Geometry check sheet. Reference: the model listing, model coordinates, mm. Face numbers are marked on the shaded views. A direction names the side the tool comes from. Round coordinates to 2 decimals unless told otherwise and drop trailing zeros. Write each loop counter-clockwise with the first axis right and the second up, starting at its lowest first coordinate (ties: lowest second). Pieces come first, ordered by that corner, then holes. Notation, with made-up numbers: (-34.5, 61.25) - (-22.5, 61.25) arc R15 ccw to (-22.5, 79.25) - close; hole circle Ø8 at (13, 28.25). An arc over 180 degrees is marked (long way). Return JSON: item names as keys, results as strings.
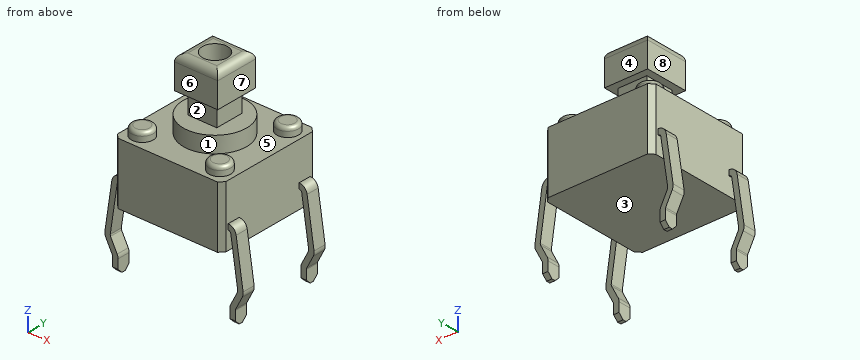
Autodesk Inventor part; units mm, degrees
ref_plane "YZ Plane" through (0, 0, 0) normal (1, 0, 0) x (0, 1, 0)
ref_plane "XZ Plane" through (0, 0, 0) normal (0, 1, 0) x (-1, 0, 0)
ref_plane "XY Plane" through (0, 0, 0) normal (0, 0, 1) x (1, 0, 0)
sketch "Sketch1" plane through (0, 0, 0) normal (0, 0, 1) x (1, 0, 0)
  line L0 (-2.75, -3) -> (2.75, -3)
  line L1 (3, -2.75) -> (3, 2.75)
  line L2 (2.75, 3) -> (-2.75, 3)
  line L3 (-3, 2.75) -> (-3, -2.75)
  line L4 (-3, -3) -> (3, 3) construction
  line L5 (3, -3) -> (-3, 3) construction
  line L6 (-2.75, 3) -> (-3, 2.75)
  line L7 (-3, -2.75) -> (-2.75, -3)
  line L8 (2.75, -3) -> (3, -2.75)
  line L9 (3, 2.75) -> (2.75, 3)
  point P0 (0, 0)
  dimension "d0" = 6
  dimension "d1" = 0.25
  dimension "d2" = 0.25
  dimension "d3" = 0.25
  dimension "d4" = 0.25
  dimension "d5" = 0.25
  dimension "d6" = 0.25
  dimension "d7" = 0.25
  dimension "d8" = 0.25
extrude "Extrusion1" add sketch "Sketch1" along normal mid plane 3.4
sketch "Sketch2" plane through (0, 0, 1.7) normal (0, 0, 1) x (1, 0, 0)
  line L0 (-2.15, -2.15) -> (2.15, -2.15) construction
  line L1 (2.15, -2.15) -> (2.15, 2.15) construction
  line L2 (2.15, 2.15) -> (-2.15, 2.15) construction
  line L3 (-2.15, 2.15) -> (-2.15, -2.15) construction
  line L4 (-2.15, -2.15) -> (2.15, 2.15) construction
  line L5 (2.15, -2.15) -> (-2.15, 2.15) construction
  circle A0 centre (-2.15, 2.15) radius 0.6
  circle A1 centre (2.15, 2.15) radius 0.6
  circle A2 centre (2.15, -2.15) radius 0.6
  circle A3 centre (-2.15, -2.15) radius 0.6
  point P0 (0, 0)
  dimension "d11" = 4.3
  dimension "d12" = 1.2
extrude "Extrusion2" add sketch "Sketch2" along normal blind 0.5
sketch "Sketch3" plane through (0, 0, 1.7) normal (0, 0, 1) x (1, 0, 0)
  circle A0 centre (0, 0) radius 1.75
  dimension "d15" = 3.5
extrude "Extrusion3" add sketch "Sketch3" along normal blind 0.9
sketch "Sketch4" plane through (0, 0, 2.6) normal (0, 0, 1) x (1, 0, 0)
  line L0 (-0.8, -0.8) -> (0.8, -0.8)
  line L1 (0.8, -0.8) -> (0.8, 0.8)
  line L2 (0.8, 0.8) -> (-0.8, 0.8)
  line L3 (-0.8, 0.8) -> (-0.8, -0.8)
  line L4 (-0.8, -0.8) -> (0.8, 0.8) construction
  line L5 (0.8, -0.8) -> (-0.8, 0.8) construction
  point P0 (0, 0)
  dimension "d18" = 1.6
extrude "Extrusion4" add sketch "Sketch4" along normal blind 1.2
sketch "Sketch5" plane through (0, 0, 3.8) normal (0, 0, 1) x (1, 0, 0)
  circle A0 centre (0, 0) radius 0.7
  line L0 (-1.2, -1.2) -> (1.2, -1.2)
  line L1 (1.2, -1.2) -> (1.2, 1.2)
  line L2 (1.2, 1.2) -> (-1.2, 1.2)
  line L3 (-1.2, 1.2) -> (-1.2, -1.2)
  line L4 (-1.2, -1.2) -> (1.2, 1.2) construction
  line L5 (1.2, -1.2) -> (-1.2, 1.2) construction
  dimension "d21" = 1.4
  dimension "d22" = 2.4
extrude "Extrusion5" add sketch "Sketch5" along normal blind 1.8
fillet "Fillet1" radius 0.4 4 edges at (0, 1.2, 5.6) (-1.2, 0, 5.6) (0, -1.2, 5.6) (1.2, 0, 5.6)
sketch "Sketch6" plane through (0, 0, 0) normal (0, 1, 0) x (-1, 0, 0)
  line L0 (-3, -1.7) -> (-3, 1.7)
  line L1 (-3, -1.7) -> (-3, 1.7)
  line L2 (-3.1484, -0.828) -> (-3.5321, -3.4214)
  arc A0 (-3.5321, -3.4214) -> (-3.5173, -3.5117) centre (-3.3838, -3.4434) ccw
  line L3 (-3.5173, -3.5117) -> (-3.1493, -4.2312)
  arc A1 (-3.1, -4.4361) -> (-3.1493, -4.2312) centre (-3.55, -4.4361) ccw
  line L4 (-3.1, -4.4361) -> (-3.1, -5.2)
  line L5 (-3.1, -5.2) -> (-3.4, -5.2)
  line L6 (-3.4, -5.2) -> (-3.4, -4.4361)
  arc A2 (-3.4, -4.4361) -> (-3.4164, -4.3678) centre (-3.55, -4.4361) ccw
  line L7 (-3.4164, -4.3678) -> (-3.7844, -3.6483)
  arc A3 (-3.8289, -3.3775) -> (-3.7844, -3.6483) centre (-3.3838, -3.4434) ccw
  line L8 (-3.8289, -3.3775) -> (-3.4452, -0.7841)
  line L9 (-3.8289, -3.3775) -> (-3.85, -3.52) construction
  line L10 (-3.85, -3.52) -> (-3.7844, -3.6483) construction
  line L11 (-3.4, -4.4361) -> (-3.4, -4.4) construction
  line L12 (-3.4, -4.4) -> (-3.4164, -4.3678) construction
  arc A4 (-3, -0.7) -> (-3.1484, -0.828) centre (-3, -0.85) ccw
  arc A5 (-3, -0.4) -> (-3.4452, -0.7841) centre (-3, -0.85) ccw
  line L13 (2.75, -1.7) -> (-2.75, -1.7)
  line L14 (0, 0) -> (0, -1.7) construction
  line L15 (-3, -0.4) -> (-3, -0.7)
  line L16 (3.1484, -0.828) -> (3.5321, -3.4214)
  arc A6 (3.5173, -3.5117) -> (3.5321, -3.4214) centre (3.3838, -3.4434) ccw
  line L17 (3.5173, -3.5117) -> (3.1493, -4.2312)
  arc A7 (3.1493, -4.2312) -> (3.1, -4.4361) centre (3.55, -4.4361) ccw
  line L18 (3.1, -4.4361) -> (3.1, -5.2)
  line L19 (3.1, -5.2) -> (3.4, -5.2)
  line L20 (3.4, -5.2) -> (3.4, -4.4361)
  arc A8 (3.4164, -4.3678) -> (3.4, -4.4361) centre (3.55, -4.4361) ccw
  line L21 (3.4164, -4.3678) -> (3.7844, -3.6483)
  arc A9 (3.7844, -3.6483) -> (3.8289, -3.3775) centre (3.3838, -3.4434) ccw
  line L22 (3.8289, -3.3775) -> (3.4452, -0.7841)
  line L23 (3.8289, -3.3775) -> (3.85, -3.52) construction
  line L24 (3.85, -3.52) -> (3.7844, -3.6483) construction
  line L25 (3.4, -4.4361) -> (3.4, -4.4) construction
  line L26 (3.4, -4.4) -> (3.4164, -4.3678) construction
  arc A10 (3.1484, -0.828) -> (3, -0.7) centre (3, -0.85) ccw
  arc A11 (3.4452, -0.7841) -> (3, -0.4) centre (3, -0.85) ccw
  line L27 (3, -0.4) -> (3, -0.7)
  dimension "d26" = 0.3
  dimension "d28" = 3.5
  dimension "d29" = 3.4
  dimension "d30" = 0.15
  dimension "d31" = 3.85
  dimension "d32" = 1.82
  dimension "d33" = 0.8
  dimension "d34" = 1
extrude "Extrusion6" add sketch "Sketch6" along normal mid plane 5.2
sketch "Sketch7" plane through (0, 0, 0) normal (0, 0, 1) x (1, 0, 0)
  line L0 (-3, 2.75) -> (-3, -2.75)
  line L1 (-4, 1.9) -> (-3, 1.9)
  line L2 (-3, 1.9) -> (-3, -1.9)
  line L3 (-3, -1.9) -> (-4, -1.9)
  line L4 (-4, -1.9) -> (-4, 1.9)
  line L5 (3, -2.75) -> (3, 2.75)
  line L6 (4, 1.9) -> (3, 1.9)
  line L7 (3, 1.9) -> (3, -1.9)
  line L8 (3, -1.9) -> (4, -1.9)
  line L9 (4, -1.9) -> (4, 1.9)
  point P0 (0, 0)
  point P1 (-3.8289, 2.6)
  point P2 (3, 0)
  point P3 (3, 0)
  point P4 (-3, 0)
  dimension "d37" = 0.7
  dimension "d40" = 1
extrude "Extrusion7" cut sketch "Sketch7" against normal through all
chamfer "Chamfer1" distance 0.25 angle 45 8 edges at (-3.25, -2.6, -5.2) (-3.25, -1.9, -5.2) (3.25, -2.6, -5.2) (3.25, -1.9, -5.2) (3.25, 1.9, -5.2) (3.25, 2.6, -5.2) (-3.25, 1.9, -5.2) (-3.25, 2.6, -5.2)
fillet "Fillet2" radius 0.2 4 edges at (-2.75, -2.15, 2.2) (1.55, -2.15, 2.2) (-2.75, 2.15, 2.2) (1.55, 2.15, 2.2)
equation "\"d2\" = d1"
equation "\"d3\" = d1"
equation "\"d4\" = d3"
equation "\"d5\" = d1"
equation "\"d6\" = d5"
equation "\"d7\" = d1"
equation "\"d8\" = d7"
equation "\"d30\" = 0.5 * d26"
properties part number "49-0005" material "ABS Plastic"
(1) Release check for a two-part mould opening along Z. For the marked faces 1, 2 and 3 record: pulls with the +Z half, pulls with the -Z half, needs draft (parallel to the pull), parting line crosses it, or undercut.
Response values:
{"face 1": "needs draft", "face 2": "undercut", "face 3": "pulls with the -Z half"}
(2) Section check B-B, the plane x = 0. Enter the section's corners in (y, z).
Response values:
{"outline": "(-3, -1.7) - (3, -1.7) - (3, 1.7) - (1.75, 1.7) - (1.75, 2.6) - (0.8, 2.6) - (0.8, 3.8) - (1.2, 3.8) - (1.2, 5.2) arc R0.4 ccw to (0.8, 5.6) - (0.7, 5.6) - (0.7, 3.8) - (-0.7, 3.8) - (-0.7, 5.6) - (-0.8, 5.6) arc R0.4 ccw to (-1.2, 5.2) - (-1.2, 3.8) - (-0.8, 3.8) - (-0.8, 2.6) - (-1.75, 2.6) - (-1.75, 1.7) - (-3, 1.7) - close"}
(3) Gauge pin test, flat ends, axial feed: pin 1 (1.1 mm diameter, centred on y = -0.5, z = 5, fed in from +X); pin 2 (1.5 mm diameter, centred on y = 2, z = -1, fed in from -X); pin 3 (0.7 mm diameter, centred on x = 0, z = 4, fed in from -Y). Record the tip position at first contact, or that the pin passes through.
Response values:
{"pin 1": "stops at x = 1.2", "pin 2": "stops at x = -3.59", "pin 3": "stops at y = -1.2"}
(4) Material ranges on line 1 along Y through (x, z) = (0, 4.4); line 2 along X through (y, z) = (-1.6, 0.5); line 3 along X through (y, z) = (0.45, 4), recorded low to high. Write a range as [from, to].
Response values:
{"line 1": "y = [-1.2, -0.7], [0.7, 1.2]", "line 2": "x = [-3, 3]", "line 3": "x = [-1.2, -0.54], [0.54, 1.2]"}
(5) Access from +Z, -Z, +X, -X, +Y, -Y to the whole of each face (thin tool, end or side, straight path). Record for the marked faces 4, 5, 6, 7 and 8.
Response values:
{"face 4": "+Z, +X, -X, +Y", "face 5": "+Z", "face 6": "+Z, +X, -X, -Y", "face 7": "+Z, +X, +Y, -Y", "face 8": "+Z, -X, +Y, -Y"}
(6) Section check C-C, the plane y = -1.05. Enter the section's corners in (x, z).
Response values:
{"outline": "(-3, -1.7) - (3, -1.7) - (3, 1.7) - (1.4, 1.7) - (1.4, 2.6) - (-1.4, 2.6) - (-1.4, 1.7) - (-3, 1.7) - close; (-1.2, 3.8) - (1.2, 3.8) - (1.2, 5.2) arc R0.4 ccw to (1.05, 5.51) - (-1.05, 5.51) arc R0.4 ccw to (-1.2, 5.2) - close"}
(7) Section check A-A, the plane z = -2.5. Enter the section's corners in (x, y), plus the area to 3 significant figures.
Response values:
{"outline": "(-3.7, -2.6) - (-3.4, -2.6) - (-3.4, -1.9) - (-3.7, -1.9) - close; (-3.7, 1.9) - (-3.4, 1.9) - (-3.4, 2.6) - (-3.7, 2.6) - close; (3.4, -2.6) - (3.7, -2.6) - (3.7, -1.9) - (3.4, -1.9) - close; (3.4, 1.9) - (3.7, 1.9) - (3.7, 2.6) - (3.4, 2.6) - close", "area": "0.849 mm^2"}
